Read the model definition and answer for the solid it produces. Units are mm, in the model's axes. Face numbers are marked on the shaded views. A direction names the side the tool comes from. Give positions to 0.01 mm unless a question says otherwise; leave off trailing zeros. Write each loop counter-clockwise with the first axis right and the second up, starting at its lowest first coordinate (ties: lowest second). Pieces come first, ordered by that corner, then holes.
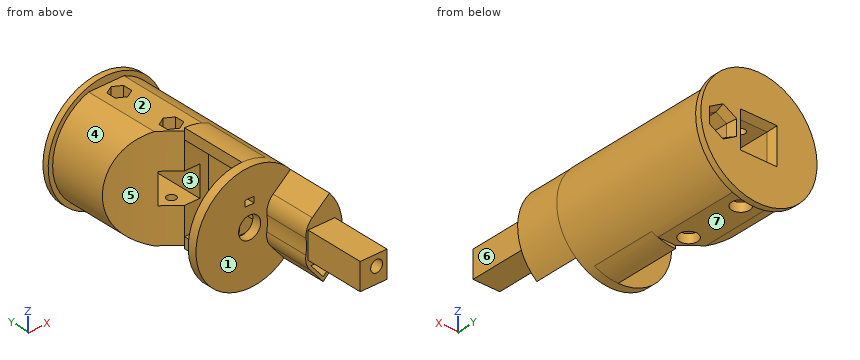
```python
from build123d import *
from build123d.topology import SkipClean

# Parameters (mm, degrees)
SKETCH_1_R          = 18
EXTRUDE_1_DEPTH     = 55
SKETCH_2_R          = 19.5
EXTRUDE_2_DEPTH     = 2
SKETCH_3_W          = 10.25
SKETCH_3_H          = 10.25
CUT_EXTRUDE_1_DEPTH = 40
EXTRUDE_3_DEPTH     = 15
SKETCH1_R           = 18
BOSS_EXTRUDE1_DEPTH = 20
SKETCH3_R           = 18
BOSS_EXTRUDE2_DEPTH = 7
SKETCH4_W           = 10.2
SKETCH4_H           = 10.2
CUT_EXTRUDE2_DEPTH  = 27
CUT_EXTRUDE4_DEPTH  = 25
BOSS_EXTRUDE3_DEPTH = 3
SKETCH9_W           = 36
SKETCH9_H           = 22
CUT_EXTRUDE5_DEPTH  = 8
SKETCH10_R          = 3.7
SKETCH10_W          = 3
SKETCH10_H          = 2
CUT_EXTRUDE6_DEPTH  = 10
SKETCH11_R          = 2
CUT_EXTRUDE7_DEPTH  = 102
SKETCH15_R          = 18
CUT_EXTRUDE9_DEPTH  = 27
CUT_EXTRUDE11_DEPTH = 30
SKETCH18_R          = 1.5
CUT_EXTRUDE12_DEPTH = 71.437916
SKETCH19_R          = 3
CUT_EXTRUDE13_DEPTH = 3
BOSS_EXTRUDE5_DEPTH = 22
CUT_EXTRUDE16_DEPTH = 4
CUT_EXTRUDE17_DEPTH = 25.4
CUT_EXTRUDE18_DEPTH = 71.437916
FILLET2_R           = 5
SKETCH30_W          = 18.8
SKETCH30_H          = 10
CUT_EXTRUDE20_DEPTH = 3
CHAMFER1_SIZE       = 1
CHAMFER1_SIZE2      = 2.747477
CHAMFER2_SIZE       = 1
CHAMFER2_SIZE2      = 2.747477
SKETCH37_W          = 9
SKETCH37_H          = 9
SKETCH37_R          = 2
BOSS_EXTRUDE7_DEPTH = 20
CUT_EXTRUDE22_DEPTH = 15
CUT_EXTRUDE23_REACH = 79.101
SKETCH40_W          = 4.363156
SKETCH40_H          = 4.363157
CUT_EXTRUDE24_DEPTH = 10
FILLET7_R           = 6


with BuildPart() as part:
    # Эскиз1 → Бобышка-Вытянуть1 (new body)
    with BuildSketch(Plane(origin=(0, 0, 0), x_dir=(1, 0, 0), z_dir=(0, 1, 0))):
        with Locations(Location((0, 0, 0), (0, 0, 270))):
            Circle(SKETCH_1_R)
    extrude(amount=EXTRUDE_1_DEPTH)

    # Эскиз2 → Бобышка-Вытянуть2 (add)
    with BuildSketch(Plane(origin=(0, 55, 0), x_dir=(1, 0, 0), z_dir=(0, 1, 0))):
        with Locations(Location((0, 0, 0), (0, 0, 270))):
            Circle(SKETCH_2_R)
    extrude(amount=EXTRUDE_2_DEPTH)

    # Эскиз3 → Вырез-Вытянуть1 (cut)
    with BuildSketch(Plane(origin=(0, 57, 0), x_dir=(1, 0, 0), z_dir=(0, 1, 0))):
        Rectangle(SKETCH_3_W, SKETCH_3_H)
    extrude(amount=-CUT_EXTRUDE_1_DEPTH, mode=Mode.SUBTRACT)

    # Эскиз4 → Бобышка-Вытянуть3 (add)
    with BuildSketch(Plane.XZ):
        with BuildLine():
            Line((5.142301, -6.128356), (11.570177, -13.7888))
            ThreePointArc((11.570177, -13.7888), (17.937391, -1.5), (13.69962, 11.675633))
            Line((13.69962, 11.675633), (5.142301, 4.382576))
            Line((5.142301, 4.382576), (5.142301, -6.128356))
        make_face()
    extrude(amount=EXTRUDE_3_DEPTH)

    # Sketch1 → Boss-Extrude1 (add)
    with BuildSketch(Plane.XZ.offset(15)):
        with Locations(Location((0, 0, 0), (0, 0, 270))):
            Circle(SKETCH1_R)
    extrude(amount=BOSS_EXTRUDE1_DEPTH)

    # Sketch3 → Boss-Extrude2 (add)
    with BuildSketch(Plane.XZ.offset(35)):
        with Locations(Location((0, 0, 0), (0, 0, 270))):
            Circle(SKETCH3_R)
    extrude(amount=BOSS_EXTRUDE2_DEPTH)

    # Sketch4 → Cut-Extrude2 (cut)
    with BuildSketch(Plane.XZ.offset(42)):
        Rectangle(SKETCH4_W, SKETCH4_H)
    extrude(amount=-CUT_EXTRUDE2_DEPTH, mode=Mode.SUBTRACT)

    # Sketch6 → Cut-Extrude4 (cut)
    with BuildSketch(Plane.XZ):
        with BuildLine():
            Line((0, 18), (0, -18))
            ThreePointArc((0, -18), (-18, 0), (0, 18))
        make_face()
    extrude(amount=-CUT_EXTRUDE4_DEPTH, mode=Mode.SUBTRACT)

    # Sketch8 → Boss-Extrude3 (add)
    with BuildSketch(Plane.XZ):
        with BuildLine():
            Line((0, -18), (0, 18))
            ThreePointArc((0, 18), (-18, 0), (0, -18))
        make_face()
    extrude(amount=-BOSS_EXTRUDE3_DEPTH)

    # Sketch9 → Cut-Extrude5 (cut)
    with BuildSketch(Plane.ZY):
        with Locations((0, 14)):
            Rectangle(SKETCH9_W, SKETCH9_H)
    extrude(amount=-CUT_EXTRUDE5_DEPTH, mode=Mode.SUBTRACT)

    # Sketch10 → Cut-Extrude6 (cut)
    with BuildSketch(Plane.XZ):
        with Locations(Location((0, 0, 0), (0, 0, 270))):
            Circle(SKETCH10_R)
        with Locations((0, 7.7)):
            Rectangle(SKETCH10_W, SKETCH10_H)
    extrude(amount=-CUT_EXTRUDE6_DEPTH, mode=Mode.SUBTRACT)

    # Sketch11 → Cut-Extrude7 (cut)
    with BuildSketch(Plane.XZ.offset(42)):
        with Locations(Location((12, 0, 0), (0, 0, 270))):
            Circle(SKETCH11_R)
    extrude(amount=-CUT_EXTRUDE7_DEPTH, mode=Mode.SUBTRACT)

    # Sketch15 → Cut-Extrude9 (cut)
    with BuildSketch(Plane.XZ.offset(42)):
        with Locations(Location((0, 0, 0), (0, 0, 310))):
            Circle(SKETCH15_R)
    extrude(amount=-CUT_EXTRUDE9_DEPTH, mode=Mode.SUBTRACT)

    # Sketch17 → Cut-Extrude11 (cut)
    with BuildSketch(Plane.XZ.offset(-25)):
        with BuildLine():
            Line((5.91608, -17), (-5.91608, -17))
            ThreePointArc((-5.91608, -17), (0, -18), (5.91608, -17))
        make_face()
        with BuildLine():
            Line((5.91608, 17), (-5.91608, 17))
            ThreePointArc((-5.91608, 17), (0, 18), (5.91608, 17))
        make_face()
    extrude(amount=-CUT_EXTRUDE11_DEPTH, mode=Mode.SUBTRACT)

    # Sketch18 → Cut-Extrude12 (cut, through all)
    with BuildSketch(Plane.XY.offset(-17)):
        with Locations(Location((0, 30, 0), (0, 0, 180))):
            Circle(SKETCH18_R)
        with Locations(Location((0, 50, 0), (0, 0, 180))):
            Circle(SKETCH18_R)
    extrude(amount=CUT_EXTRUDE12_DEPTH, mode=Mode.SUBTRACT)

    # Sketch19 → Cut-Extrude13 (cut)
    with BuildSketch(Plane.XY.offset(-17)):
        with Locations((0, 30)):
            Circle(SKETCH19_R)
        with Locations((0, 50)):
            Circle(SKETCH19_R)
    extrude(amount=CUT_EXTRUDE13_DEPTH, mode=Mode.SUBTRACT)

    # Sketch23 → Boss-Extrude5 (add)
    with BuildSketch(Plane(origin=(0, 3, 0), x_dir=(1, 0, 0), z_dir=(0, 1, 0))):
        with BuildLine():
            Line((0, -14.4), (8, -14.4))
            Line((8, -14.4), (8, -16.124515))
            ThreePointArc((8, -16.124515), (4.10845, -17.524858), (0, -18))
            Line((0, -18), (0, -14.4))
        make_face()
        with BuildLine():
            Line((0, 14.4), (8, 14.4))
            Line((8, 14.4), (8, 16.124515))
            ThreePointArc((8, 16.124515), (4.10845, 17.524858), (0, 18))
            Line((0, 18), (0, 14.4))
        make_face()
    extrude(amount=BOSS_EXTRUDE5_DEPTH)

    # Sketch25 → Cut-Extrude16 (cut)
    with BuildSketch(Plane.XY.offset(17)):
        Polygon((2.771281, 28.4), (2.771281, 31.6), (0, 33.2), (-2.771281, 31.6), (-2.771281, 28.4), (0, 26.8), align=None)
        Polygon((-2.782127, 48.418934), (-0.02182, 46.800074), (2.760307, 48.38114), (2.782127, 51.581066), (0.02182, 53.199926), (-2.760307, 51.61886), align=None)
    extrude(amount=-CUT_EXTRUDE16_DEPTH, mode=Mode.SUBTRACT)

    # Sketch26 → Cut-Extrude17 (cut)
    with BuildSketch(Plane(origin=(0, 57, 0), x_dir=(1, 0, 0), z_dir=(0, 1, 0))):
        Polygon((8.449296, -2.05), (12, -4.1), (15.550704, -2.05), (15.550704, 2.05), (12, 4.1), (8.449296, 2.05), align=None)
    extrude(amount=-CUT_EXTRUDE17_DEPTH, mode=Mode.SUBTRACT)

    # Sketch27 → Cut-Extrude18 (cut, through all)
    with BuildSketch(Plane.XY.offset(17)):
        with BuildLine():
            Line((-20, 36.547005), (-20, 25))
            Line((-20, 25), (0, 25))
            ThreePointArc((0, 25), (-9.324199, 31.944024), (-20, 36.547005))
        make_face()
    extrude(amount=-CUT_EXTRUDE18_DEPTH, mode=Mode.SUBTRACT)

    # Fillet2
    fillet2_edges = [part.edges().sort_by_distance(p)[0] for p in [
        (8, 14, -14.4),
        (8, 14, 14.4),
    ]]
    fillet(fillet2_edges, radius=FILLET2_R)

    # Sketch30 → Cut-Extrude20 (cut)
    with BuildSketch(Plane.ZY.offset(-8)):
        with Locations((0, 8)):
            Rectangle(SKETCH30_W, SKETCH30_H)
    extrude(amount=-CUT_EXTRUDE20_DEPTH, mode=Mode.SUBTRACT)

    # Chamfer1
    chamfer1_edges = [part.edges().sort_by_distance(p)[0] for p in [
        (5.125, 57, 0),
        (0, 57, -5.125),
        (-5.125, 57, 0),
        (0, 57, 5.125),
    ]]
    chamfer1_side = [part.faces().sort_by_distance(p)[0] for p in [
        (0, 57, -18.948457),
    ]]
    chamfer(chamfer1_edges, length=CHAMFER1_SIZE, length2=CHAMFER1_SIZE2, reference=chamfer1_side[0])

    # Chamfer2
    chamfer2_edges = [part.edges().sort_by_distance(p)[0] for p in [
        (8.449296, 57, 0),
        (10.224648, 57, 3.075),
        (13.775352, 57, 3.075),
        (15.550704, 57, 0),
        (13.775352, 57, -3.075),
        (10.224648, 57, -3.075),
    ]]
    chamfer2_side = [part.faces().sort_by_distance(p)[0] for p in [
        (6.676543, 57, 0),
    ]]
    chamfer(chamfer2_edges, length=CHAMFER2_SIZE, length2=CHAMFER2_SIZE2, reference=chamfer2_side[0])

    # Sketch37 → Boss-Extrude7 (add)
    with SkipClean():  # the faces are left unmerged after this step: merging them gives an invalid solid
        with BuildSketch(Plane.XZ.offset(15)):
            with Locations((10.978823, -0.87289)):
                Rectangle(SKETCH37_W, SKETCH37_H)
            with Locations(Location((12, 0, 0), (0, 0, 270))):
                Circle(SKETCH37_R, mode=Mode.SUBTRACT)
        extrude(amount=BOSS_EXTRUDE7_DEPTH)

    # Sketch38 → Cut-Extrude22 (cut)
    with SkipClean():  # the faces are left unmerged after this step: merging them gives an invalid solid
        with BuildSketch(Plane.XZ.offset(15)):
            with BuildLine():
                Line((5.142301, -6.128356), (5.142301, 4.382576))
                ThreePointArc((5.142301, 4.382576), (5.978823, -0.87289), (5.142301, -6.128356))
            make_face()
        extrude(amount=-CUT_EXTRUDE22_DEPTH, mode=Mode.SUBTRACT)

    # Cut-Extrude23: up to this face of the body (flat: up to its plane)
    cut_extrude23_end = Plane(part.part.faces().sort_by_distance((9.45036, 13, 0))[0])
    # Sketch39 → Cut-Extrude23 (cut, up to the picked face)
    with BuildSketch(Plane.XZ.offset(15), mode=Mode.PRIVATE) as cut_extrude23_sk1:
        with BuildLine():
            Line((7.420734, -7.37289), (15.420734, -7.37289))
            ThreePointArc((15.420734, -7.37289), (13.728515, -10.030416), (11.598853, -12.352179))
            Line((11.598853, -12.352179), (7.420734, -7.37289))
        make_face()
    cut_extrude23_tool1 = split(extrude(cut_extrude23_sk1.sketch, amount=-CUT_EXTRUDE23_REACH, mode=Mode.PRIVATE), bisect_by=cut_extrude23_end, keep=Keep.BOTH, mode=Mode.PRIVATE)
    add(cut_extrude23_tool1.solids().sort_by(Axis((11.596211, -15, -9.081847), (0, 1, 0)))[0], mode=Mode.SUBTRACT)

    # Sketch40 → Cut-Extrude24 (cut)
    with SkipClean():  # the faces are left unmerged after this step: merging them gives an invalid solid
        with BuildSketch(Plane(origin=(0, 3, 0), x_dir=(1, 0, 0), z_dir=(0, 1, 0))):
            with Locations((9.602312, 9.554468)):
                Rectangle(SKETCH40_W, SKETCH40_H)
        extrude(amount=CUT_EXTRUDE24_DEPTH, mode=Mode.SUBTRACT)

    # Fillet7
    fillet7_edges = [part.edges().sort_by_distance(p)[0] for p in [
        (5.142301, -7.5, 4.382576),
        (5.142301, -7.5, -6.128356),
    ]]
    fillet(fillet7_edges, radius=FILLET7_R)


solid = part.part
```
Item 1: Section D-D (x = -7) is taken. Write down the section's boundary in (y, z), and give its area (3 significant figures).
Result set:
outline: (0, -16.58) - (3, -16.58) - (3, 16.58) - (0, 16.58) - close; (30.52, -16.58) - (55, -16.58) - (55, -18.2) - (57, -18.2) - (57, 18.2) - (55, 18.2) - (55, 16.58) - (30.52, 16.58) - close
area: 984 mm2
Item 2: Section C-C (y = 50) is taken. Give the number of separate pieces and of enclosed holes in the cut face, and give its area (3 significant figures).
Result set:
separate pieces: 2
enclosed holes: 1
area: 763 mm2
Item 3: Determine the mould class of the marked faces 1, 2 and 3 for opening direction Y: pulls with the +Y half, pulls with the -Y half, needs draft (parallel to the pull), parting line crosses it, or undercut.
Result set:
face 1: pulls with the -Y half
face 2: undercut
face 3: needs draft
Item 4: Find the intervals of material crossed by line 1 along Z through (x, y) = (2, 29.5) (3 decimals); line 2 along Z through (x, y) = (11.5, 0.5); line 3 along Y through (x, z) = (0, 9), in increasing order.
Result set:
line 1: z = -14 to -5.125, 5.125 to 13
line 2: z = -13.85 to -12.23, -7.37 to -1.94, 1.94 to 13.85
line 3: y = 0 to 3, 25 to 28.5, 31.5 to 48.5, 51.5 to 57
Item 5: Which of the six approach directions +Z, -Z, +X, -X, +Y, -Y give full straight-line access (tool end or side, diameter ignored) to the marked faces 4, 5, 6 and 7?
Result set:
face 4: -X, -Y
face 5: +Z, -Z, -X
face 6: +Z, -Z, +X, -Y
face 7: -Z, +X, -X
Item 6: Section B-B (x = -17) is taken. Write down the section's boundary in (y, z).
Result set:
outline: (0, -5.92) - (3, -5.92) - (3, 5.92) - (0, 5.92) - close; (35.55, -5.92) - (55, -5.92) - (55, -9.55) - (57, -9.55) - (57, 9.55) - (55, 9.55) - (55, 5.92) - (35.55, 5.92) - close
Item 7: Each of these flat-tipped pins is pushed along its axis until it touches: pin 1 Ø12 at (x, y) = (9.5, -1) entering from -Z; pin 2 Ø4.5 at (y, z) = (39.5, -1) entering from +X; pin 3 Ø1.8 at (x, y) = (9, 7) entering from +Z. Where does it stop, or does it pass through?
Result set:
pin 1: stops at z = -17.64
pin 2: stops at x = 18
pin 3: stops at z = 16.07
Item 8: Section A-A (y = 21.5) is taken. Write down the section's boundary in (x, z), and give its area (3 significant figures).
Result set:
outline: (0, -18) arc R18 ccw to (8, -16.12) arc R18 ccw to (8, 16.12) arc R18 ccw to (0, 18) - (0, 14.4) - (3, 14.4) arc R5 cw to (8, 9.4) - (8, -9.4) arc R5 cw to (3, -14.4) - (0, -14.4) - close; hole circle Ø4 at (12, 0)
area: 277 mm2
